```python
from build123d import *

# Parameters (mm, degrees)
BOSS_EXTRUDE3_DEPTH   = 12
CUT_EXTRUDE5_DEPTH    = 2
SKETCH12_R            = 2.5
CUT_EXTRUDE6_DEPTH    = 11
SKETCH13_R            = 5.5
CUT_EXTRUDE7_DEPTH    = 5
SKETCH16_R            = 11
SKETCH16_R_2          = 5.5
BOSS_EXTRUDE4_DEPTH   = 2
FILLET3_R             = 1
FILLET4_R             = 0.5
M3_TAPPED_HOLE1_D     = 2.5
M3_TAPPED_HOLE1_DEPTH = 7.5
M3_TAPPED_HOLE1_TIP   = 0.751075774
CHAMFER1_SIZE         = 0.3


with BuildPart() as part:
    # Sketch10 → Boss-Extrude3 (new body)
    with BuildSketch(Plane(origin=(0, 0, 0), x_dir=(1, 0, 0), z_dir=(0, 1, 0))):
        Polygon((-21.15, 17.15), (-17.15, 21.15), (17.15, 21.15), (21.15, 17.15), (21.15, -17.15), (17.15, -21.15), (-17.15, -21.15), (-21.15, -17.15), align=None)
    extrude(amount=BOSS_EXTRUDE3_DEPTH)

    # Sketch11 → Cut-Extrude5 (cut)
    with BuildSketch(Plane(origin=(0, 12, 0), x_dir=(1, 0, 0), z_dir=(0, 1, 0))):
        Polygon((-14.15, -21.15), (14.15, -21.15), (21.15, -14.15), (21.15, 14.15), (14.15, 21.15), (-14.15, 21.15), (-21.15, 14.15), (-21.15, -14.15), align=None)
    extrude(amount=-CUT_EXTRUDE5_DEPTH, mode=Mode.SUBTRACT)

    # Sketch12 → Cut-Extrude6 (cut, through all)
    with BuildSketch(Plane(origin=(0, 10, 0), x_dir=(1, 0, 0), z_dir=(0, 1, 0))):
        Circle(SKETCH12_R)
    extrude(amount=-CUT_EXTRUDE6_DEPTH, mode=Mode.SUBTRACT)

    # Sketch13 → Cut-Extrude7 (cut)
    with BuildSketch(Plane.XZ):
        Circle(SKETCH13_R)
    extrude(amount=-CUT_EXTRUDE7_DEPTH, mode=Mode.SUBTRACT)

    # Sketch16 → Boss-Extrude4 (add)
    with BuildSketch(Plane.XZ):
        Circle(SKETCH16_R)
        Circle(SKETCH16_R_2, mode=Mode.SUBTRACT)
    extrude(amount=BOSS_EXTRUDE4_DEPTH)

    # Fillet3
    fillet3_edges = [part.edges().sort_by_distance(p)[0] for p in [
        (-19.15, 0, -19.15),
        (0, 0, -21.15),
        (19.15, 0, -19.15),
        (21.15, 0, 0),
        (19.15, 0, 19.15),
        (0, 0, 21.15),
        (-19.15, 0, 19.15),
        (-21.15, 0, 0),
    ]]
    fillet(fillet3_edges, radius=FILLET3_R)

    # Fillet4
    fillet4_edges = [part.edges().sort_by_distance(p)[0] for p in [
        (-11, 0, 0),
        (-11, -2, 0),
        (-5.5, -2, 0),
    ]]
    fillet(fillet4_edges, radius=FILLET4_R)

    # M3 Tapped Hole1
    with Locations(Plane(origin=(0, 0, 0), x_dir=(-1, 0, 0), z_dir=(0, -1, 0))):
        with Locations((-15.5, -15.5), (15.5, -15.5), (15.5, 15.5), (-15.5, 15.5)):
            Hole(M3_TAPPED_HOLE1_D / 2, depth=M3_TAPPED_HOLE1_DEPTH)
            with Locations((0, 0, -(M3_TAPPED_HOLE1_DEPTH + M3_TAPPED_HOLE1_TIP / 2))):  # 118° drill point
                Cone(0, M3_TAPPED_HOLE1_D / 2, M3_TAPPED_HOLE1_TIP, mode=Mode.SUBTRACT)

    # Chamfer1
    chamfer1_edges = [part.edges().sort_by_distance(p)[0] for p in [
        (14.25, 0, -15.5),
        (-16.75, 0, -15.5),
        (-16.75, 0, 15.5),
        (14.25, 0, 15.5),
    ]]
    chamfer(chamfer1_edges, length=CHAMFER1_SIZE)


solid = part.part
```
CAD build for the part. Positions are in the model's coordinates, mm. A direction names the side the tool comes from. Round coordinates to 2 decimals unless told otherwise and drop trailing zeros. Order: outer loops, then holes, each group sorted by start corner. A loop starts at its lowest first (then second) coordinate and runs counter-clockwise, first axis right, second up. Notation, with made-up numbers: (54.5, 43) -> (60.5, 43) arc R32 ccw to (60.5, 73) -> close; hole circle Ø6 at (-8, 62.5). An arc over 180 degrees is marked (long way). Write item = value, one per line.
(1) Cut at A-A (z = 0). Write the cut outline in (x, y).
Answers follow:
outline = (-21.15, 1) arc R1 ccw to (-20.15, 0) -> (-11.5, 0) arc R0.5 cw to (-11, -0.5) -> (-11, -1.5) arc R0.5 ccw to (-10.5, -2) -> (-6, -2) arc R0.5 ccw to (-5.5, -1.5) -> (-5.5, 5) -> (-2.5, 5) -> (-2.5, 10) -> (-21.15, 10) -> close; (2.5, 5) -> (5.5, 5) -> (5.5, -1.5) arc R0.5 ccw to (6, -2) -> (10.5, -2) arc R0.5 ccw to (11, -1.5) -> (11, -0.5) arc R0.5 cw to (11.5, 0) -> (20.15, 0) arc R1 ccw to (21.15, 1) -> (21.15, 10) -> (2.5, 10) -> close
(2) Cut at C-C (y = 9.25). Write the cut outline in (x, z).
Answers follow:
outline = (-21.15, -17.15) -> (-17.15, -21.15) -> (17.15, -21.15) -> (21.15, -17.15) -> (21.15, 17.15) -> (17.15, 21.15) -> (-17.15, 21.15) -> (-21.15, 17.15) -> close; hole circle Ø5 at (0, 0)
(3) 3-axis set-ups, long thin cutter, end or side, ignore diameter. For faces 4 (the cylindrical face through (-20.865, 0.301, -0.24)), 5 (the cylindrical face through (14.579, 3.95, -16.345)), 6 (the flat face through (4, 10, 0)): which of +Z, -Z, +X, -X, +Y, -Y reach the whole face in a straight line?
Answers follow:
face_4 = +Z, -Z, -X, -Y
face_5 = -Y
face_6 = +Y
(4) Flat gauge pins, fed straight in: P1, Ø3, axis at x = 15.5, z = -15.5, coming from the +Y side; P2, Ø1, axis at x = 15.5, z = -13.5, coming from the -Y side; P3, Ø5.5, axis at x = -0.5, z = 2, coming from the -Y side. Where does each tip first touch, or does it go through?
Answers follow:
P1 = 10
P2 = 0
P3 = 5
(5) Cut at B-B (y = 3.25). Write the cut outline in (x, z).
Answers follow:
outline = (-21.15, -17.15) -> (-17.15, -21.15) -> (17.15, -21.15) -> (21.15, -17.15) -> (21.15, 17.15) -> (17.15, 21.15) -> (-17.15, 21.15) -> (-21.15, 17.15) -> close; hole circle Ø2.5 at (-15.5, -15.5); hole circle Ø2.5 at (-15.5, 15.5); hole circle Ø11 at (0, 0); hole circle Ø2.5 at (15.5, -15.5); hole circle Ø2.5 at (15.5, 15.5)
(6) Pull direction X, two halves, no side cores. Call faces 1 (the flat face through (-17.6, 11, -17.7)), 2 (the cylindrical face through (-0.24, 0.301, 20.865)), 3 (the cylindrical face through (18.92, 0.301, 18.976)): +X half, -X half, draft (parallel to the pull), parting line (faces both ways), or undercut.
Answers follow:
face_1 = undercut
face_2 = draft
face_3 = +X half
(7) Cut at D-D (y = 7). Write the cut outline in (x, z), plus the area to 3 significant figures.
Answers follow:
outline = (-21.15, -17.15) -> (-17.15, -21.15) -> (17.15, -21.15) -> (21.15, -17.15) -> (21.15, 17.15) -> (17.15, 21.15) -> (-17.15, 21.15) -> (-21.15, 17.15) -> close; hole circle Ø2.5 at (-15.5, -15.5); hole circle Ø2.5 at (-15.5, 15.5); hole circle Ø5 at (0, 0); hole circle Ø2.5 at (15.5, -15.5); hole circle Ø2.5 at (15.5, 15.5)
area = 1,720 mm²
(8) Drill centre lines: L1, parallel to Z at x = 15.5, y = 2.5; L2, parallel to Z at x = 0, y = 6.1. Where is each one in solid material? Low to high.
Answers follow:
L1 = -21.15 to -16.75, -14.25 to 14.25, 16.75 to 21.15
L2 = -21.15 to -2.5, 2.5 to 21.15
